Check sheet for the modelled part. Datum: model origin and axes. Units: mm. A direction names the side the tool comes from. Coordinates: 2 decimals unless noted, no trailing zeros. Write each loop counter-clockwise with the first axis right and the second up, starting at its lowest first coordinate (ties: lowest second). Pieces come first, ordered by that corner, then holes. Notation, with made-up numbers: M 28.5,62.5 L 37.5,62.5 A18 cw 37.5,96.5 Z; hole C 63.25,15 d1. An arc over 180 degrees is marked long. Answer as CSV lines item,"result". Start each with the question number.
Q1. Sectioned sample at C-C, the plane y = 17.5. Record the cut outline in (x, z), then the cut area to 3 significant figures.
Q2. Access from +Z, -Z, +X, -X, +Y, -Y to the whole of each face (thin tool, end or side, straight path). Record for faces 4 (the cylindrical face through (-9.94, 20.97, 13.01)), 5 (the flat face through (-32.48, 17, -10)), 6 (the flat face through (-12.48, 18, 0)).
Q3. Mould release check, pull along Y, two halves, no side actions. Record for faces 1 (the flat face through (-20, 17, 17.5)), 2 (the cylindrical face through (-22.62, 17.95, 13.98)), 3 (the flat face through (-20, 0, 0)): pulls with the +Y half, pulls with the -Y half, needs draft (parallel to the pull), parting line crosses it, or undercut.
Q4. Sectioned sample at B-B, the plane x = -26.5. Record the cut outline in (y, z).
Q5. Depth check by flat-ended pin: pin 1 Ø2.5 at (y, z) = (17.5, -12.55) entering from +X; pin 2 Ø10 at (y, z) = (19.5, -1.5) entering from -X; pin 3 Ø4 at (y, z) = (27.5, 2.5) entering from -X; pin 4 Ø3.5 at (y, z) = (16.5, 13) entering from +X. Enter the tip coordinate at first touch or a pass-through.
Q6. Sectioned sample at A-A, the plane z = 12.55. Record the cut outline in (x, y), then the cut area to 3 significant figures.
Q7. Thickness scan on line 1 along Y through (x, z) = (-26.25, -12.55); line 2 along Y through (x, z) = (-10.5, -12.55); line 3 along X through (y, z) = (17, 14.5). Record the ranges inside material, lowest first. Write a range as from..to.
Q8. Sectioned sample at D-D, the plane x = -19.25. Record the cut outline in (y, z).
from build123d import *

# Parameters (mm, degrees)
BOSS_EXTRUDE1_DEPTH = 35
SKETCH3_R           = 6.3
CUT_EXTRUDE1_DEPTH  = 20
SKETCH4_R           = 1.5
CUT_EXTRUDE2_DEPTH  = 47.435439128
SKETCH5_R           = 3.5
CUT_EXTRUDE3_DEPTH  = 5


with BuildPart() as part:
    # Sketch1 → Boss-Extrude1 (new body)
    with BuildSketch(Plane(origin=(0, 0, 0), x_dir=(1, 0, 0), z_dir=(0, 1, 0))):
        with BuildLine():
            Line((-32.48, -7.6), (-32.48, -17.5))
            Line((-32.48, -17.5), (-7.48, -17.5))
            Line((-7.48, -17.5), (-7.48, 17.5))
            Line((-7.48, 17.5), (-32.48, 17.5))
            Line((-32.48, 17.5), (-32.48, 7.6))
            ThreePointArc((-32.48, 7.6), (-24.88, 0), (-32.48, -7.6))
        make_face()
    extrude(amount=BOSS_EXTRUDE1_DEPTH)

    # Sketch3 → Cut-Extrude1 (cut)
    with BuildSketch(Plane.ZY.offset(32.48)):
        with Locations((0, 17.5)):
            Circle(SKETCH3_R)
    extrude(amount=-CUT_EXTRUDE1_DEPTH, mode=Mode.SUBTRACT)

    # Sketch4 → Cut-Extrude2 (cut, through all)
    with BuildSketch(Plane.ZY.offset(32.48)):
        with Locations((12.55, 17.5)):
            Circle(SKETCH4_R)
        with Locations((-12.55, 17.5)):
            Circle(SKETCH4_R)
    extrude(amount=-CUT_EXTRUDE2_DEPTH, mode=Mode.SUBTRACT)

    # Sketch5 → Cut-Extrude3 (cut)
    with BuildSketch(Plane(origin=(-7.48, 0, 0), x_dir=(0, 0, -1), z_dir=(1, 0, 0))):
        with Locations((-12.55, 17.5)):
            Circle(SKETCH5_R)
        with Locations((12.55, 17.5)):
            Circle(SKETCH5_R)
    extrude(amount=-CUT_EXTRUDE3_DEPTH, mode=Mode.SUBTRACT)


solid = part.part
Output:
1,outline,"M -32.48,-17.5 L -7.48,-17.5 L -7.48,-16.05 L -12.48,-16.05 L -12.48,-14.05 L -32.48,-14.05 Z; M -32.48,-11.05 L -12.48,-11.05 L -12.48,-9.05 L -7.48,-9.05 L -7.48,9.05 L -12.48,9.05 L -12.48,11.05 L -32.48,11.05 L -32.48,7.6 A7.6 cw -28.23,6.3 L -12.48,6.3 L -12.48,-6.3 L -28.23,-6.3 A7.6 cw -32.48,-7.6 Z; M -32.48,14.05 L -12.48,14.05 L -12.48,16.05 L -7.48,16.05 L -7.48,17.5 L -32.48,17.5 Z"
1,area,"425 mm^2"
2,face 4,"+X"
2,face 5,"+Z, -Z, -X, +Y, -Y"
2,face 6,"-X"
3,face 1,"needs draft"
3,face 2,"undercut"
3,face 3,"pulls with the -Y half"
4,outline,"M 0,-17.5 L 35,-17.5 L 35,-4.69 L 21.71,-4.69 A6.3 cw 13.29,-4.69 L 0,-4.69 Z; M 0,4.69 L 13.29,4.69 A6.3 cw 21.71,4.69 L 35,4.69 L 35,17.5 L 0,17.5 Z; hole C 17.5,-12.55 d3; hole C 17.5,12.55 d3"
5,pin 1,"passes through"
5,pin 2,"stops at x = -28.54"
5,pin 3,"stops at x = -26.36"
5,pin 4,"stops at x = -12.48"
6,outline,"M -32.48,0 L -7.48,0 L -7.48,14 L -12.48,14 L -12.48,16 L -32.48,16 Z; M -32.48,19 L -12.48,19 L -12.48,21 L -7.48,21 L -7.48,35 L -32.48,35 Z"
6,area,"780 mm^2"
7,line 1,"y = 0..16, 19..35"
7,line 2,"y = 0..14, 21..35"
7,line 3,"x = -32.48..-12.48"
8,outline,"M 0,-17.5 L 35,-17.5 L 35,17.5 L 0,17.5 Z; hole C 17.5,0 d12.6; hole C 17.5,-12.55 d3; hole C 17.5,12.55 d3"
